from build123d import *

# Parameters (mm, degrees)
BOSS_EXTRUDE1_DEPTH          = 20
M10_TAPPED_HOLE1_D           = 8.5
M10_TAPPED_HOLE1_DEPTH       = 27.5
M10_TAPPED_HOLE1_CSINK_D     = 10.05
M10_TAPPED_HOLE1_CSINK_ANGLE = 90
M10_TAPPED_HOLE1_TIP         = 2.553657631
M8_TAPPED_HOLE1_D            = 6.8
M8_TAPPED_HOLE1_DEPTH        = 22.25
M8_TAPPED_HOLE1_CSINK_D      = 8.05
M8_TAPPED_HOLE1_CSINK_ANGLE  = 90
M8_TAPPED_HOLE1_TIP          = 2.042926105
CUT_EXTRUDE1_DEPTH           = 72.576963501
SKETCH7_R                    = 21.448918638
SKETCH7_R_2                  = 10.5
CUT_EXTRUDE2_DEPTH           = 9
FILLET1_R                    = 5


with BuildPart() as part:
    # Sketch1 → Boss-Extrude1 (new body)
    with BuildSketch(Plane(origin=(0, 0, 0), x_dir=(0, 0, -1), z_dir=(1, 0, 0))):
        with BuildLine():
            Line((-35.65, 0), (35.65, 0))
            Line((35.65, 0), (35.65, -49.098))
            Line((35.65, -49.098), (23.65, -49.098))
            ThreePointArc((23.65, -49.098), (0, -25.448), (-23.65, -49.098))
            Line((-23.65, -49.098), (-35.65, -49.098))
            Line((-35.65, -49.098), (-48.09, -49.098))
            Line((-48.09, -49.098), (-48.09, 0))
            Line((-48.09, 0), (-35.65, 0))
        make_face()
    extrude(amount=BOSS_EXTRUDE1_DEPTH)

    # M10 Tapped Hole1
    with Locations(Plane(origin=(0, 0, 0), x_dir=(1, 0, 0), z_dir=(0, 1, 0))):
        with Locations((10, -38.09), (10, 25.65)):
            CounterSinkHole(M10_TAPPED_HOLE1_D / 2, M10_TAPPED_HOLE1_CSINK_D / 2, depth=M10_TAPPED_HOLE1_DEPTH, counter_sink_angle=M10_TAPPED_HOLE1_CSINK_ANGLE)
            with Locations((0, 0, -(M10_TAPPED_HOLE1_DEPTH + M10_TAPPED_HOLE1_TIP / 2))):  # 118° drill point
                Cone(0, M10_TAPPED_HOLE1_D / 2, M10_TAPPED_HOLE1_TIP, mode=Mode.SUBTRACT)

    # M8 Tapped Hole1
    with Locations(Plane(origin=(0, -49.098, 0), x_dir=(-1, 0, 0), z_dir=(0, -1, 0))):
        with Locations((-10, -35.87), (-10, 29.65)):
            CounterSinkHole(M8_TAPPED_HOLE1_D / 2, M8_TAPPED_HOLE1_CSINK_D / 2, depth=M8_TAPPED_HOLE1_DEPTH, counter_sink_angle=M8_TAPPED_HOLE1_CSINK_ANGLE)
            with Locations((0, 0, -(M8_TAPPED_HOLE1_DEPTH + M8_TAPPED_HOLE1_TIP / 2))):  # 118° drill point
                Cone(0, M8_TAPPED_HOLE1_D / 2, M8_TAPPED_HOLE1_TIP, mode=Mode.SUBTRACT)

    # Sketch6 → Cut-Extrude1 (cut, through all)
    with BuildSketch(Plane(origin=(20, 0, 0), x_dir=(0, 0, -1), z_dir=(1, 0, 0))):
        with BuildLine():
            Line((13.78, 0.1), (13.78, -0.1))
            ThreePointArc((13.78, -0.1), (-6.22, -20.1), (-26.22, -0.1))
            Line((-26.22, -0.1), (-26.22, 0.1))
            ThreePointArc((-26.22, 0.1), (-6.22, 20.1), (13.78, 0.1))
        make_face()
    extrude(amount=-CUT_EXTRUDE1_DEPTH, mode=Mode.SUBTRACT)

    # Sketch7 → Cut-Extrude2 (cut)
    with BuildSketch(Plane.XZ.offset(49.098)):
        with Locations((10, 35.87)):
            Circle(SKETCH7_R)
        with Locations((10, 35.87)):
            Circle(SKETCH7_R_2, mode=Mode.SUBTRACT)
    extrude(amount=-CUT_EXTRUDE2_DEPTH, mode=Mode.SUBTRACT)

    # Fillet1
    fillet1_edges = [part.edges().sort_by_distance(p)[0] for p in [
        (10, -40.098, 21.870585269),
    ]]
    fillet(fillet1_edges, radius=FILLET1_R)


solid = part.part
Design review of the part built by this model. Coordinates are the model's own, in mm. A direction names the side the tool comes from. Round coordinates to 2 decimals unless told otherwise and drop trailing zeros. Write each loop counter-clockwise with the first axis right and the second up, starting at its lowest first coordinate (ties: lowest second). Pieces come first, ordered by that corner, then holes. Notation, with made-up numbers: M 42.25,-17.75 L 88.25,-17.75 A20 cw 88.25,-10.75 Z; hole C 17,-9 d4. An arc over 180 degrees is marked long. One line per item, written item: value. Start each with the question number.
1. Clearance check with flat-ended pins moving along their axes: P1, Ø9, axis at x = 10, z = 35.87, coming from the -Y side; P2, Ø10, axis at y = -43.5, z = 16, coming from the -X side; P3, Ø12, axis at x = 18, z = 4, coming from the -Y side. State where each tip first meets the part, or that it passes through.
2. Take a section at A-A on y = -14.5. State the section outline as (x, z) points, then the cut area to 3 significant figures.
3. Take a section at D-D on y = -7.5. State the section outline as (x, z) points.
4. Draft analysis for pull direction Z (two halves, no side actions). For faces 5 (the face through (9.81, -44.66, 25.37)), 6 (the face through (10, -20, 48.09)), 7 (the face through (20, -24, 6)), state which applies: pulls with the +Z half, pulls with the -Z half, needs draft (parallel to the pull), parting line crosses it, or undercut.
5. For faces 1 (the face through (11.828, -37.509, -32.517)), 2 (the face through (9.86, -39.393, 22.436)), 3 (the face through (10, -40.098, 47)), 4 (the face through (10, -49.098, -34)), list the 3-axis set-ups (+Z, -Z, +X, -X, +Y, -Y) from which the entire face can be reached by the end or side of a thin tool; tool diameter is ignored.
6. Take a section at B-B on y = -22. State the section outline as (x, z) points.
7. To check wall thickness, follow probe 1 along Z at (x, y) = (10, -43.5); probe 2 along Z at (x, y) = (10, -13); probe 3 along X at (y, z) = (-36.5, -29.65). State the ranges of each line that lie inside material, in increasing order. Write a range as from..to.
8. Take a section at C-C on z = -19.5. State the section outline as (x, y) points.
Computed:
1. P1: stops at y = -49.1
1. P2: passes through
1. P3: stops at y = -27.67
2. outline: M 0,-35.65 L 20,-35.65 L 20,-7.66 L 0,-7.66 Z; M 0,20.1 L 20,20.1 L 20,48.09 L 0,48.09 Z; hole C 10,-25.65 d8.5; hole C 10,38.09 d8.5
2. area: 1,010 mm²
3. outline: M 0,-35.65 L 20,-35.65 L 20,-12.36 L 0,-12.36 Z; M 0,24.8 L 20,24.8 L 20,48.09 L 0,48.09 Z; hole C 10,-25.65 d8.5; hole C 10,38.09 d8.5
4. face 5: undercut
4. face 6: pulls with the +Z half
4. face 7: needs draft
5. face 1: -Y
5. face 2: +X, -X, -Y
5. face 3: +Z, -Y
5. face 4: +Z, -Z, +X, -X, -Y
6. outline: M 0,-35.65 L 20,-35.65 L 20,48.09 L 0,48.09 Z; hole C 10,-25.65 d8.5; hole C 10,38.09 d8.5
7. probe 1: z = -35.65..-33.05, -26.25..-22.98, 25.37..32.47, 39.27..46.37
7. probe 2: z = -35.65..-29.9, -21.4..-9.06, 21.5..33.84, 42.34..48.09
7. probe 3: x = 0..6.6, 13.4..20
8. outline: M 0,-35.72 L 20,-35.72 L 20,0 L 0,0 Z
